Verification items for the finished model (mm, model axes). A direction names the side the tool comes from. Give positions to 0.01 mm unless a question says otherwise; leave off trailing zeros. Write each loop counter-clockwise with the first axis right and the second up, starting at its lowest first coordinate (ties: lowest second). Pieces come first, ordered by that corner, then holes. Notation, with made-up numbers: (38.25, 29) - (90.25, 29) arc R30 cw to (90.25, 67) - close; hole circle Ø4 at (25, 68). An arc over 180 degrees is marked (long way). Put each result on its own line as item: value.
from build123d import *

# Parameters (mm, degrees)
F0_W     = 38.1
F0_H     = 50.8
F1_DEPTH = 6.35
F2_R     = 3.175
F3_DEPTH = 6.351
F4_W     = 3.175
F4_H     = 15.490544
F4_H_2   = 14.951406
F5_DEPTH = 6.351
F6_W     = 6.35
F6_H     = 14.951406
F7_DEPTH = 6.351


with BuildPart() as f1:
    # F0 (on Right) → F1 (new body)
    with BuildSketch(Plane.YZ):
        with Locations((-0.666162, 1.42497)):
            Rectangle(F0_W, F0_H)
    extrude(amount=F1_DEPTH)

    # F2 (on face) → F3 (cut, through all)
    with BuildSketch(Plane.YZ.offset(6.35)):
        with Locations((0, 17.93497)):
            Circle(F2_R)
    extrude(amount=-F3_DEPTH, mode=Mode.SUBTRACT)

    # F4 (on face) → F5 (cut, through all)
    with BuildSketch(Plane.YZ.offset(6.35)):
        with Locations((-18.128662, -16.229758)):
            Rectangle(F4_W, F4_H)
        with Locations((16.796338, -16.499327)):
            Rectangle(F4_W, F4_H_2)
    extrude(amount=-F5_DEPTH, mode=Mode.SUBTRACT)

    # F6 (on face) → F7 (cut, through all)
    with BuildSketch(Plane.YZ.offset(6.35)):
        with Locations((0, -16.499327)):
            Rectangle(F6_W, F6_H)
    extrude(amount=-F7_DEPTH, mode=Mode.SUBTRACT)


solid = f1.part
Q1. Section check A-A, the plane y = 0. Record the cut outline in (x, z), plus the area to 3 significant figures.
Answers follow:
outline: (0, -9.02) - (6.35, -9.02) - (6.35, 14.76) - (0, 14.76) - close; (0, 21.11) - (6.35, 21.11) - (6.35, 26.82) - (0, 26.82) - close
area: 187 mm2
Q2. Set-up check for faces 4 (the face through (3, -18, -8.484)), 5 (the face through (3.219, -0.413, 21.083)), 6 (the face through (3, 15.209, -17)), 7 (the face through (3, -3.175, -17)): record each of +Z, -Z, +X, -X, +Y, -Y from which the full face is reachable in a straight line by a thin tool's end or side.
Answers follow:
face 4: -Z, +X, -X, -Y
face 5: +X, -X
face 6: -Z, +X, -X, +Y
face 7: -Z, +X, -X
Q3. Section check C-C, the plane x = 5. Record the cut outline in (y, z) (3 decimals), plus the area to 3 significant figures.
Answers follow:
outline: (-19.716, -8.484) - (-16.541, -8.484) - (-16.541, -23.975) - (-3.175, -23.975) - (-3.175, -9.024) - (3.175, -9.024) - (3.175, -23.975) - (15.209, -23.975) - (15.209, -9.024) - (18.384, -9.024) - (18.384, 26.825) - (-19.716, 26.825) - close; hole circle Ø6.35 at (0, 17.935)
area: 1,710 mm2
Q4. Scan lines: line 1 along Z through (x, y) = (4.25, 0); line 2 along Y through (x, z) = (4.75, -22) (3 decimals); line 3 along Z through (x, y) = (4.5, 2). Record each from-to range of solid material in increasing order.
Answers follow:
line 1: z = -9.02 to 14.76, 21.11 to 26.82
line 2: y = -16.541 to -3.175, 3.175 to 15.209
line 3: z = -9.02 to 15.47, 20.4 to 26.82
Q5. Go/stop test with flat-tipped pins: pin 1 Ø1 at (x, y) = (2.5, 17.5) entering from -Z; pin 2 Ø1.9 at (x, z) = (3.5, -18.5) entering from +Y; pin 3 Ø5 at (y, z) = (7, 15) entering from -X; pin 4 Ø1 at (x, y) = (3, -19) entering from -Z. Record where each tip stops, or that it passes through.
Answers follow:
pin 1: stops at z = -9.02
pin 2: stops at y = 15.21
pin 3: stops at x = 0
pin 4: stops at z = -8.48
Q6. Section check B-B, the plane z = 16. Record the cut outline in (x, y).
Answers follow:
outline: (0, -19.72) - (6.35, -19.72) - (6.35, -2.52) - (0, -2.52) - close; (0, 2.52) - (6.35, 2.52) - (6.35, 18.38) - (0, 18.38) - close
Q7. Release check for a two-part mould opening along Y. For faces 1 (the face through (3, -19.716, 9)), 2 (the face through (3, 3.175, -17)), 3 (the face through (0, -1, 2)) record: released by +Y, released by -Y, zero draft, split by the parting line, or undercut.
Answers follow:
face 1: released by -Y
face 2: undercut
face 3: zero draft
